```python
from build123d import *

# Parameters (mm, degrees)
F1_DEPTH = 12
F2_R     = 2.5
F2_R_2   = 3
F3_DEPTH = 25


with BuildPart() as f1:
    # F0 (on Front) → F1 (new body)
    with BuildSketch(Plane.XZ):
        Polygon((20.467626, 11.379912), (-24.532374, 11.379912), (-24.532374, -0.620088), (50.467626, -0.620088), (50.467626, 1.879912), align=None)
    extrude(amount=F1_DEPTH)

    # F2 (on face) → F3 (cut)
    with BuildSketch(Plane.XY.offset(11.379912)):
        with Locations((-16.532374, -6)):
            Circle(F2_R)
        with Locations((13.467626, -6)):
            Circle(F2_R_2)
    extrude(amount=-F3_DEPTH, mode=Mode.SUBTRACT)


solid = f1.part
```
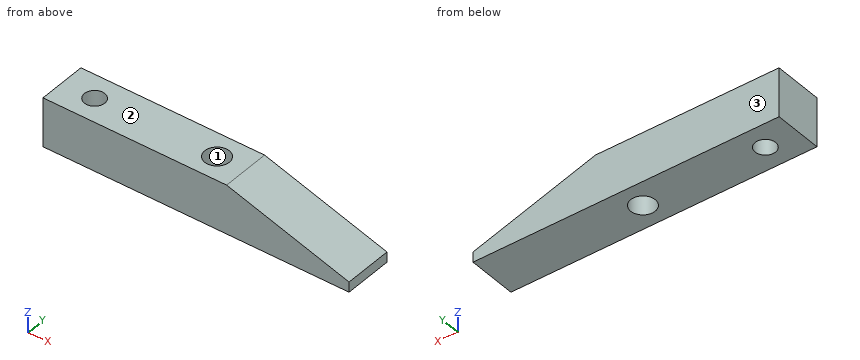
Here's how the part is built. I have some questions about the finished solid (model axes, mm). Face numbers are marked on the shaded views. Coordinates: 2 decimals unless noted, no trailing zeros. Order: outer loops, then holes, each group sorted by start corner. A loop starts at its lowest first (then second) coordinate and runs counter-clockwise, first axis right, second up. Notation, with made-up numbers: (83.25, 51) - (108.25, 51) arc R8 cw to (108.25, 60) - close; hole circle Ø1 at (-31.75, 78.25). An arc over 180 degrees is marked (long way). One line per question, with ' | ' between items.
(1) If we mould it in two halves opening along Y, with no side actions, what happens to the marked faces 1, 2 and 3? For each: pulls with the +Y half, pulls with the -Y half, needs draft (parallel to the pull), parting line crosses it, or undercut.
Report:
face 1: undercut | face 2: needs draft | face 3: pulls with the +Y half
(2) Will this pin go through, and if not, where does the flat tip stop? pin 1 (6.5 mm diameter, centred on x = -16.53, y = -6, fed in from +Z).
Report:
pin 1: stops at z = 11.38
(3) Suppose I cut it at A-A on y = -6. List the corners of the cut face in (x, z) for me.
Report:
outline: (-24.53, -0.62) - (-19.03, -0.62) - (-19.03, 11.38) - (-24.53, 11.38) - close; (-14.03, -0.62) - (10.47, -0.62) - (10.47, 11.38) - (-14.03, 11.38) - close; (16.47, -0.62) - (50.47, -0.62) - (50.47, 1.88) - (20.47, 11.38) - (16.47, 11.38) - close
(4) Suppose I cut it at B-B on y = -1.75. List the corners of the cut face in (x, z) for me.
Report:
outline: (-24.53, -0.62) - (50.47, -0.62) - (50.47, 1.88) - (20.47, 11.38) - (-24.53, 11.38) - close
(5) Suppose I cut it at C-C on z = 4.5. List the corners of the cut face in (x, y) for me, and give its area (3 significant figures).
Report:
outline: (-24.53, -12) - (42.19, -12) - (42.19, 0) - (-24.53, 0) - close; hole circle Ø5 at (-16.53, -6); hole circle Ø6 at (13.47, -6) | area: 753 mm2
(6) If I drill on L1, parallel to Y at x = -16.5, z = 4; L2, parallel to Y at x = 15.5, z = 6.5; L3, parallel to Z at x = 38, y = -8, over which ranges is the centre line in solid material (lowest first)?
Report:
L1: y = -12 to -8.5, -3.5 to 0 | L2: y = -12 to -8.21, -3.79 to 0 | L3: z = -0.62 to 5.83
